The listing builds one solid part. Answer for the finished solid, in the listing's coordinates (mm). Give positions to 0.01 mm unless a question says otherwise; leave off trailing zeros. Loops run counter-clockwise (first coordinate to the right, second up) from the corner with the lowest first, then second, coordinate; pieces in that order, holes last. Notation, with made-up numbers: (-10.5, -28) - (4.5, -28) arc R7 ccw to (4.5, -23) - close; hole circle Ø1 at (-35.75, 53). An arc over 180 degrees is marked (long way). Write each question's results on one line, items separated by ' | '.
from build123d import *

# Parameters (mm, degrees)
SKETCH1_W                       = 25
SKETCH1_H                       = 812.8
BOSS_EXTRUDE1_DEPTH             = 3
CUT_EXTRUDE4_DEPTH              = 10
F_1_4_0_25_DIAMETER_HOLE1_D     = 6.35
F_1_4_0_25_DIAMETER_HOLE1_DEPTH = 5.84
F_1_4_0_25_DIAMETER_HOLE1_TIP   = 1.907732465


with BuildPart() as part:
    # Sketch1 → Boss-Extrude1 (new body)
    with BuildSketch(Plane.XY):
        Rectangle(SKETCH1_W, SKETCH1_H)
    extrude(amount=BOSS_EXTRUDE1_DEPTH)

    # Sketch5 → Cut-Extrude4 (cut)
    with BuildSketch(Plane.XY.offset(3)):
        with BuildLine():
            Line((2.5, 125.980140029), (22.5, 125.980140029))
            ThreePointArc((22.5, 125.980140029), (25.5, 122.980140029), (22.5, 119.980140029))
            Line((22.5, 119.980140029), (2.5, 119.980140029))
            ThreePointArc((2.5, 119.980140029), (-0.5, 122.980140029), (2.5, 125.980140029))
        make_face()
        with BuildLine():
            Line((2.5, 97.480140029), (22.5, 97.480140029))
            ThreePointArc((22.5, 97.480140029), (25.5, 94.480140029), (22.5, 91.480140029))
            Line((22.5, 91.480140029), (2.5, 91.480140029))
            ThreePointArc((2.5, 91.480140029), (-0.5, 94.480140029), (2.5, 97.480140029))
        make_face()
        with BuildLine():
            Line((2.5, -262.629859971), (22.5, -262.629859971))
            ThreePointArc((22.5, -262.629859971), (25.5, -265.629859971), (22.5, -268.629859971))
            Line((22.5, -268.629859971), (2.5, -268.629859971))
            ThreePointArc((2.5, -268.629859971), (-0.5, -265.629859971), (2.5, -262.629859971))
        make_face()
        with BuildLine():
            Line((2.5, -291.129859971), (22.5, -291.129859971))
            ThreePointArc((22.5, -291.129859971), (25.5, -294.129859971), (22.5, -297.129859971))
            Line((22.5, -297.129859971), (2.5, -297.129859971))
            ThreePointArc((2.5, -297.129859971), (-0.5, -294.129859971), (2.5, -291.129859971))
        make_face()
    extrude(amount=-CUT_EXTRUDE4_DEPTH, mode=Mode.SUBTRACT)

    # 1/4 (0.25) Diameter Hole1
    with Locations(Plane.XY.offset(3)):
        with Locations((0, 393.7), (0, -393.7)):
            Hole(F_1_4_0_25_DIAMETER_HOLE1_D / 2, depth=F_1_4_0_25_DIAMETER_HOLE1_DEPTH)
            with Locations((0, 0, -(F_1_4_0_25_DIAMETER_HOLE1_DEPTH + F_1_4_0_25_DIAMETER_HOLE1_TIP / 2))):  # 118° drill point
                Cone(0, F_1_4_0_25_DIAMETER_HOLE1_D / 2, F_1_4_0_25_DIAMETER_HOLE1_TIP, mode=Mode.SUBTRACT)


solid = part.part
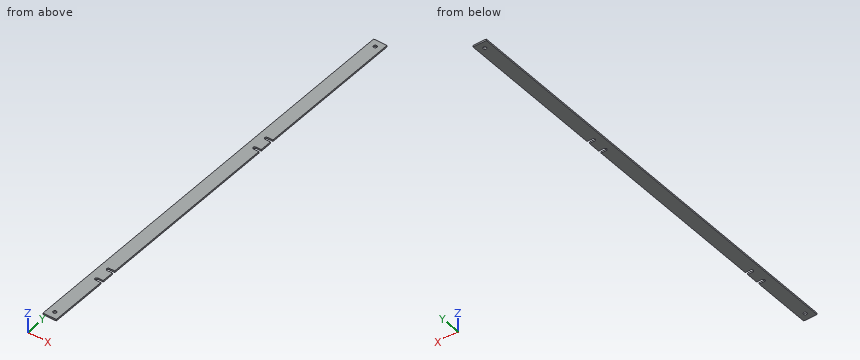
Item 1: A cutting plane is placed at A-A, the plane x = 7.25. Determine the outline of the cut face in (y, z).
Values found:
outline: (-406.4, 0) - (-297.13, 0) - (-297.13, 3) - (-406.4, 3) - close; (-291.13, 0) - (-268.63, 0) - (-268.63, 3) - (-291.13, 3) - close; (-262.63, 0) - (91.48, 0) - (91.48, 3) - (-262.63, 3) - close; (97.48, 0) - (119.98, 0) - (119.98, 3) - (97.48, 3) - close; (125.98, 0) - (406.4, 0) - (406.4, 3) - (125.98, 3) - close
Item 2: A cutting plane is placed at B-B, the plane z = 1.5. Determine the outline of the cut face in (x, y) (3 decimals).
Values found:
outline: (-12.5, -406.4) - (12.5, -406.4) - (12.5, -297.13) - (2.5, -297.13) arc R3 cw to (2.5, -291.13) - (12.5, -291.13) - (12.5, -268.63) - (2.5, -268.63) arc R3 cw to (2.5, -262.63) - (12.5, -262.63) - (12.5, 91.48) - (2.5, 91.48) arc R3 cw to (2.5, 97.48) - (12.5, 97.48) - (12.5, 119.98) - (2.5, 119.98) arc R3 cw to (2.5, 125.98) - (12.5, 125.98) - (12.5, 406.4) - (-12.5, 406.4) - close; hole circle Ø6.35 at (0, -393.7); hole circle Ø6.35 at (0, 393.7)
Item 3: A flat-ended cylindrical pin translates along its axis: P1, Ø5, axis at x = 0, y = 393.7, coming from the -Z side. Find the tip coordinate at first contact, or state that the pin passes through.
Values found:
P1: passes through
Item 4: Find the intervals of material crossed by line 1 along Y through (x, z) = (10.75, 0.4); line 2 along Y through (x, z) = (-1, 2.4); line 3 along X through (y, z) = (-393.7, 1.5) (3 decimals), in increasing order. Write a range as [from, to].
Values found:
line 1: y = [-406.4, -297.13], [-291.13, -268.63], [-262.63, 91.48], [97.48, 119.98], [125.98, 406.4] | line 2: y = [-406.4, -396.71], [-390.69, 390.69], [396.71, 406.4] | line 3: x = [-12.5, -3.175], [3.175, 12.5]
